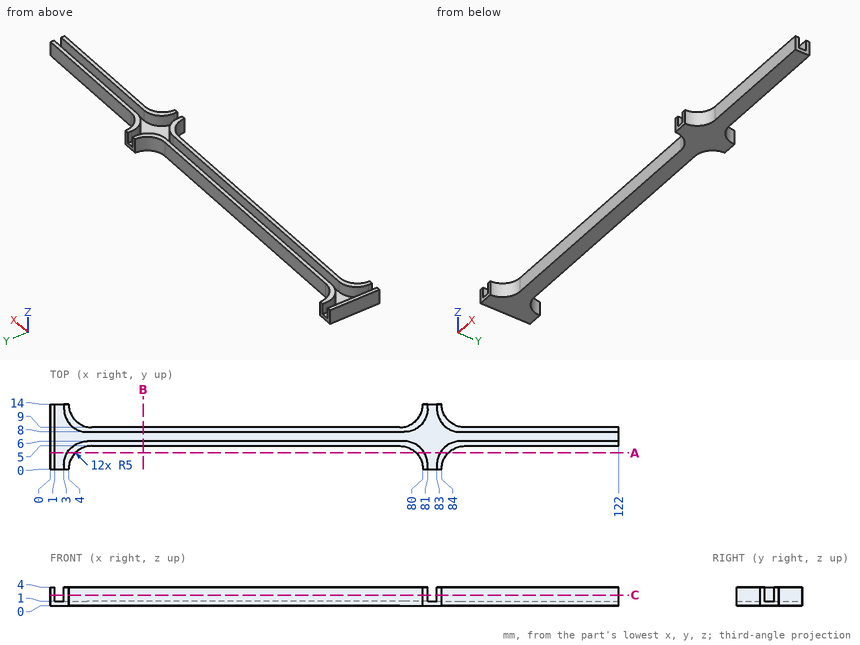
Could you check a few things on this drawing? It's one solid part, dimensions in mm from its lowest x, y, z. Give positions to 0.01 mm unless a question says otherwise; leave off trailing zeros. Order: outer loops, then holes, each group sorted by start corner. A loop starts at its lowest first (then second) coordinate and runs counter-clockwise, first axis right, second up.
1. Suppose I cut it at A-A (y = 3.5). Write out the boundary of the cut face in (x, z).
Answers below:
outline: (0, 0) - (5.43, 0) - (5.43, 4) - (3.67, 4) - (3.67, 1) - (1, 1) - (1, 4) - (0, 4) - close; (78.57, 0) - (85.43, 0) - (85.43, 4) - (83.67, 4) - (83.67, 1) - (80.33, 1) - (80.33, 4) - (78.57, 4) - close
2. For pin 1 (0.5 mm diameter, centred on y = 13.5, z = 2.5, fed in from +X); pin 2 (2 mm diameter, centred on x = 46, z = 2, fed in from -Y); pin 3 (6 mm diameter, centred on x = 25.5, y = 2.5, fed in from +Z); pin 4 (0.9 mm diameter, centred on x = 98, z = 2.5, fed in from +Y), each with a flat end and sliding along its axis, tell me the tip position at first contact or that it passes through.
Answers below:
pin 1: stops at x = 84.06
pin 2: stops at y = 5
pin 3: stops at z = 4
pin 4: stops at y = 9
3. Suppose I cut it at C-C (z = 2.3). State how many separate pieces and enclosed holes the cut face has, plus the area to 3 significant figures.
Answers below:
separate pieces: 5
enclosed holes: 0
area: 278 mm2
4. Suppose I cut it at B-B (x = 20). Write out the boundary of the cut face in (y, z), plus the area to 3 significant figures.
Answers below:
outline: (5, 0) - (9, 0) - (9, 4) - (8, 4) - (8, 1) - (6, 1) - (6, 4) - (5, 4) - close
area: 10.0 mm2
5. I need wall thicknesses on L1, parallel to Y at x = 75, z = 1.15; L2, parallel to X at y = 4, z = 3.75; L3, parallel to X at y = 1, z = 1.75. Which ranges of each line are inside material? Lowest first, please.
Answers below:
L1: y = 5 to 6, 8 to 9
L2: x = 0 to 1, 4 to 6, 78 to 80, 84 to 86
L3: x = 0 to 1, 3 to 4.1, 79.9 to 81, 83 to 84.1
